Autodesk Inventor part; units mm, degrees
ref_plane "YZ Plane" through (0, 0, 0) normal (1, 0, 0) x (0, 1, 0)
ref_plane "XZ Plane" through (0, 0, 0) normal (0, 1, 0) x (-1, 0, 0)
ref_plane "XY Plane" through (0, 0, 0) normal (0, 0, 1) x (1, 0, 0)
sketch "Skizze1" plane through (0, 0, 0) normal (0, 0, 1) x (1, 0, 0)
  line L0 (-12, 25) -> (12, 25)
  line L1 (12, 25) -> (12, -25)
  line L2 (12, -25) -> (-12, -25)
  line L3 (-12, -25) -> (-12, 25)
  line L4 (-16.8, 0) -> (16.8, 0)
  line L5 (0, -35) -> (0, 35)
  point P0 (0, 0)
  dimension "d0" = 24
  dimension "d1" = 50
extrude "Extrusion1" add sketch "Skizze1" along normal blind 15
sketch "Skizze2" plane through (0, 0, 15) normal (0, 0, 1) x (1, 0, 0)
  line L0 (-16.8, 0) -> (16.8, 0)
  line L1 (0, -35) -> (0, 35)
  line L2 (-8, 7.5) -> (8, 7.5)
  line L3 (8, 7.5) -> (8, -7.5)
  line L4 (8, -7.5) -> (-8, -7.5)
  line L5 (-8, -7.5) -> (-8, 7.5)
  point P0 (0, 0)
  dimension "d4" = 16
  dimension "d5" = 15
hole "Bohrung1" at (-8, 7.5, 15) at (8, 7.5, 15) at (8, -7.5, 15) at (-8, -7.5, 15) direction (0, 0, -1) diameter 3.242 end through all
sketch "Skizze3" plane through (0, 0, 15) normal (0, 0, 1) x (1, 0, 0)
  circle A0 centre (0, 15) radius 2.75
  circle A1 centre (0, -15) radius 2.75
  point P0 (0, 0)
hole "Bohrung2" at (0, 15, 15) at (0, -15, 15) direction (0, 0, -1) diameter 4.134 end through all
properties part number "13_0204_029"
Check sheet for the modelled part. Datum: model origin and axes. Units: mm. Round coordinates to 2 decimals unless told otherwise and drop trailing zeros. Order: outer loops, then holes, each group sorted by start corner. A loop starts at its lowest first (then second) coordinate and runs counter-clockwise, first axis right, second up. Notation, with made-up numbers: M 80,32 L 91,32 A22 cw 91,40 Z; hole C 42,24.5 d10. An arc over 180 degrees is marked long. Answer in a Markdown table with one row per item.
(1) Gauge pin test, flat ends, axial feed: pin 1 (3 mm diameter, centred on x = 8, y = -7.5, fed in from -Z); pin 2 (3 mm diameter, centred on x = 4, y = -15.5, fed in from -Z). Record the tip position at first contact, or that the pin passes through.
Findings:
| item | result |
|---|---|
| pin 1 | passes through |
| pin 2 | stops at z = 0 |
(2) Section check C-C on z = 13.5. Record the boundary of the cut face in (x, y), plus the area to 3 significant figures.
Findings:
| item | result |
|---|---|
| outline | M -12,-25 L 12,-25 L 12,25 L -12,25 Z; hole C -8,-7.5 d3.24; hole C -8,7.5 d3.24; hole C 0,-15 d4.13; hole C 0,15 d4.13; hole C 8,-7.5 d3.24; hole C 8,7.5 d3.24 |
| area | 1,140 mm^2 |
(3) Draft check along Y on faces 1 (the flat face through (0, 25, 7)), 2 (the cylindrical face through (0.79, 13.09, 7.4)), 3 (the flat face through (0, 0, 0)). Enter one of: +Y half, -Y half, draft (parallel to the pull), parting line (faces both ways), or undercut.
Findings:
| item | result |
|---|---|
| face 1 | +Y half |
| face 2 | undercut |
| face 3 | draft |
(4) Section check B-B on x = -8. Record the boundary of the cut face in (y, z), plus the area to 3 significant figures.
Findings:
| item | result |
|---|---|
| outline | M -25,0 L -9.12,0 L -9.12,15 L -25,15 Z; M -5.88,0 L 5.88,0 L 5.88,15 L -5.88,15 Z; M 9.12,0 L 25,0 L 25,15 L 9.12,15 Z |
| area | 653 mm^2 |
(5) Material ranges on line 1 along X through (y, z) = (-7.5, 9.5); line 2 along Y through (x, z) = (8, 12); line 3 along Y through (x, z) = (0, 5.75), recorded low to high. Write a range as from..to.
Findings:
| item | result |
|---|---|
| line 1 | x = -12..-9.62, -6.38..6.38, 9.62..12 |
| line 2 | y = -25..-9.12, -5.88..5.88, 9.12..25 |
| line 3 | y = -25..-17.07, -12.93..12.93, 17.07..25 |
(6) Section check D-D on y = 15. Record the boundary of the cut face in (x, z).
Findings:
| item | result |
|---|---|
| outline | M -12,0 L -2.07,0 L -2.07,15 L -12,15 Z; M 2.07,0 L 12,0 L 12,15 L 2.07,15 Z |
(7) Section check A-A on y = -7.5. Record the boundary of the cut face in (x, z), plus the area to 3 significant figures.
Findings:
| item | result |
|---|---|
| outline | M -12,0 L -9.62,0 L -9.62,15 L -12,15 Z; M -6.38,0 L 6.38,0 L 6.38,15 L -6.38,15 Z; M 9.62,0 L 12,0 L 12,15 L 9.62,15 Z |
| area | 263 mm^2 |
